```python
from build123d import *

# Parameters (mm, degrees)
IZIM1_W                     = 60
IZIM1_H                     = 40
IZIM1_W_2                   = 56
IZIM1_H_2                   = 36
Y_KSEKLIK_EKSTR_ZYON1_DEPTH = 500
KES_EKSTR_ZYON1_DEPTH       = 700


with BuildPart() as part:
    # Çizim1 → Yükseklik-Ekstrüzyon1 (new body)
    with BuildSketch(Plane(origin=(0, 0, 0), x_dir=(1, 0, 0), z_dir=(0, 1, 0))):
        with Locations((30, 20)):
            Rectangle(IZIM1_W, IZIM1_H)
        with Locations((30, 20)):
            Rectangle(IZIM1_W_2, IZIM1_H_2, mode=Mode.SUBTRACT)
    extrude(amount=Y_KSEKLIK_EKSTR_ZYON1_DEPTH)

    # Çizim2 → Kes-Ekstrüzyon1 (cut)
    with BuildSketch(Plane(origin=(0, 0, -40), x_dir=(-1, 0, 0), z_dir=(0, 0, -1))):
        Polygon((-60, 440), (0, 500), (-60, 500), align=None)
        Polygon((-60, 0), (0, 0), (-60, 60), align=None)
    extrude(amount=-KES_EKSTR_ZYON1_DEPTH, mode=Mode.SUBTRACT)


solid = part.part
```
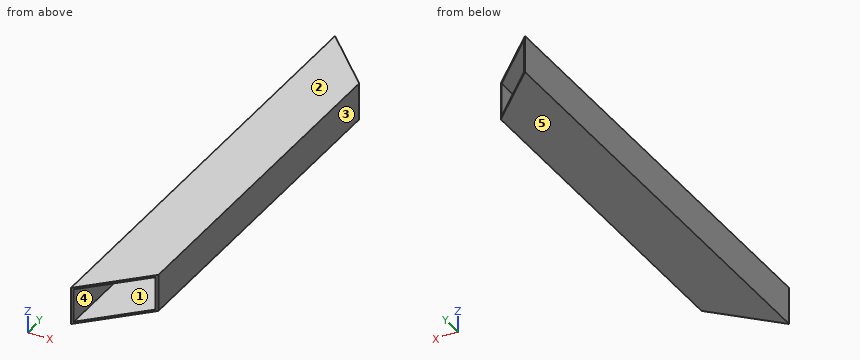
Source: CAD feature listing. Evaluate the final solid. Frame: model axes, mm. Face numbers are marked on the shaded views. A direction names the side the tool comes from. Give positions to 0.01 mm unless a question says otherwise; leave off trailing zeros. Loops run counter-clockwise (first coordinate to the right, second up) from the corner with the lowest first, then second, coordinate; pieces in that order, holes last. Notation, with made-up numbers: (39, 6.25) -> (84, 6.25) arc R25 cw to (84, 36.25) -> close; hole circle Ø7 at (14.25, 28). An arc over 180 degrees is marked (long way). Use a Markdown table: item, result. Add a question column.
(1) Ray query, line 1 (Z direction, x = 48, y = 276); line 2 (X direction, y = 100.5, z = -36); line 3 (X direction, y = 53, z = -27.5). Return the intervals inside material, ascending.
(2) Pull-direction query (Z, two-part tool) for the marked faces 1, 2 and 3; classes: +Z half, -Z half, draft (parallel to the pull), parting line (faces both ways), or undercut.
(3) First-contact query: pin 1 Ø12 at (x, z) = (26, -5) entering from -Y; pin 2 Ø10 at (x, z) = (37, -35) entering from -Y. Flat tips, straight axial feed; report the tip coordinate or a pass-through.
(4) Section query C-C (z = -13). Output: boundary loops of the cut face in (x, y).
(5) Section query A-A (x = 25). Output: boundary loops of the cut face in (y, z), then the cut area to 3 significant figures.
(6) Section query B-B (y = 279). Output: boundary loops of the cut face in (x, z), then the cut area to 3 significant figures.
(7) Access query for the marked faces 4 and 5. Directions: +Z, -Z, +X, -X, +Y, -Y. A direction counts if a zero-diameter tool reaches every point of the face in a straight line with its end or side. Return the directions, or none.
Checked values:
| question | item | result |
|---|---|---|
| 1 | line 1 | -40 to -38, -2 to 0 |
| 1 | line 2 | 0 to 2, 58 to 60 |
| 1 | line 3 | 0 to 2 |
| 2 | face 1 | undercut |
| 2 | face 2 | +Z half |
| 2 | face 3 | draft |
| 3 | pin 1 | y = 20.8 |
| 3 | pin 2 | y = 33 |
| 4 | outline | (0, 0) -> (2, 2) -> (2, 498) -> (0, 500) -> close; (58, 58) -> (60, 60) -> (60, 440) -> (58, 442) -> close |
| 5 | outline | (25, -40) -> (475, -40) -> (475, -38) -> (25, -38) -> close; (25, -2) -> (475, -2) -> (475, 0) -> (25, 0) -> close |
| 5 | area | 1,800 mm^2 |
| 6 | outline | (0, -40) -> (60, -40) -> (60, 0) -> (0, 0) -> close; hole (2, -38) -> (58, -38) -> (58, -2) -> (2, -2) -> close |
| 6 | area | 384 mm^2 |
| 7 | face 4 | +Y, -Y |
| 7 | face 5 | -Z, +X, -X, +Y, -Y |
